Geometry: final body of the model. Coordinates: model frame, mm. A direction names the side the tool comes from. Give positions to 0.01 mm unless a question says otherwise; leave off trailing zeros. Write each loop counter-clockwise with the first axis right and the second up, starting at its lowest first coordinate (ties: lowest second). Pieces come first, ordered by that corner, then holes. Notation, with made-up numbers: M 67.5,-33.5 L 112.5,-33.5 A25 cw 112.5,1.5 Z; hole C -3,28 d11. An arc over 180 degrees is marked long. Use a Markdown table: item, result. Add a question column.
(1) Pin query (flat end, axial travel): pin 1 Ø1.5 at (y, z) = (-2, -14) entering from +X; pin 2 Ø1.5 at (x, y) = (-9.5, -1) entering from +Z; pin 3 Ø1.5 at (x, z) = (-1, -37.5) entering from -Y. Return the tip coordinate at first contact, or that it passes through.
(2) Cut plane C-C (z = -17.5). Output: boundary loops of the cut face in (x, y), plus the area to 3 significant figures.
(3) Cut plane A-A (x = -11.25). Output: boundary loops of the cut face in (y, z), plus the area to 3 significant figures.
(4) Reachability of faces 4 (the flat face through (-4, 3, -25)), 5 (the flat face through (5, 1, -20)), 6 (the flat face through (4, 0, -25)) from +Z, -Z, +X, -X, +Y, -Y: full face, straight path, thin tool, end or side. Return the list, or none.
(5) Cut plane D-D (x = 6.5). Output: boundary loops of the cut face in (y, z), plus the area to 3 significant figures.
(6) Material intervals for L1, parallel to Z at x = 6, y = 1.15; L2, parallel to X at y = 1.55, z = -43.5; L3, parallel to Z at x = -10.75, y = -1.9, sorted ascending.
(7) Cut plane B-B (y = -1.65). Output: boundary loops of the cut face in (x, z).
(8) Draft query along Z for faces 1 (the flat face through (-7, 1, -50)), 2 (the flat face through (-18, 0, -25)), 3 (the flat face through (5, 1, -42)). Return one class per face: released by +Z, released by -Z, zero draft, split by the parting line, or undercut.
Autodesk Inventor part; units mm, degrees
ref_plane "YZ Plane" through (0, 0, 0) normal (1, 0, 0) x (0, 1, 0)
ref_plane "XZ Plane" through (0, 0, 0) normal (0, 1, 0) x (-1, 0, 0)
ref_plane "XY Plane" through (0, 0, 0) normal (0, 0, 1) x (1, 0, 0)
sketch "Sketch1" plane through (0, 0, 0) normal (0, 1, 0) x (-1, 0, 0)
  line L0 (0, 0) -> (0, -50)
  line L1 (0, -50) -> (-10, -50)
  line L2 (-10, -50) -> (-10, 0)
  line L3 (-10, 0) -> (0, 0)
  line L4 (-5, -50) -> (-5, -46)
  line L5 (-5, -46) -> (-3, -46)
  line L6 (-3, -46) -> (-3, -42)
  line L7 (-3, -42) -> (-7, -42)
  line L8 (-7, -42) -> (-7, -46)
  line L9 (-7, -46) -> (-5, -46)
  line L10 (-5, -42) -> (-5, -33)
  line L11 (-5, -33) -> (-7, -33)
  line L12 (-7, -33) -> (-7, -29)
  line L13 (-7, -29) -> (-3, -29)
  line L14 (-3, -29) -> (-3, -33)
  line L15 (-5, -33) -> (-3, -33)
  line L16 (-5, -29) -> (-5, -20)
  line L17 (-5, -20) -> (-3, -20)
  line L18 (-3, -20) -> (-3, -16)
  line L19 (-3, -16) -> (-7, -16)
  line L20 (-7, -16) -> (-7, -20)
  line L21 (-5, -20) -> (-7, -20)
  line L22 (-5, -16) -> (-5, -7)
  line L23 (-5, -7) -> (-7, -7)
  line L24 (-7, -7) -> (-7, -3)
  line L25 (-7, -3) -> (-3, -3)
  line L26 (-5, -7) -> (-3, -7)
  line L27 (-3, -7) -> (-3, -3)
  line L28 (0, -50) -> (2, -50)
  line L29 (2, -50) -> (2, 0)
  line L30 (2, 0) -> (0, 0)
  dimension "d0" = 50
  dimension "d1" = 10
  dimension "d2" = 90
  dimension "d3" = 4
  dimension "d4" = 2
  dimension "d5" = 4
  dimension "d6" = 4
  dimension "d7" = 9
  dimension "d8" = 4
  dimension "d9" = 9
  dimension "d10" = 4
  dimension "d11" = 9
  dimension "d12" = 4
  dimension "d13" = 2
extrude "Extrusion1" add sketch "Sketch1" along normal blind 3
sketch "Sketch2" plane through (-2, 0, -50) normal (-1, 0, 0) x (0, 0, 1)
  line L0 (0, 0) -> (0, 3)
  line L1 (0, 3) -> (50, 3)
  line L2 (50, 3) -> (50, -3)
  line L3 (50, -3) -> (0, -3)
  line L4 (0, -3) -> (0, 3)
  point P0 (50, 0)
  dimension "d16" = 6
extrude "Extrusion2" add sketch "Sketch2" along normal blind 16
sketch "Sketch3" plane through (0, 3, 0) normal (0, 1, 0) x (1, 0, 0)
  line L0 (-2, 0) -> (-18, 0)
  line L1 (-10, 0) -> (-10, 50)
  line L2 (10, 50) -> (-18, 50)
  line L3 (-12.5, 41.5) -> (-7.5, 41.5)
  line L4 (-7.5, 41.5) -> (-7.5, 46.5)
  line L5 (-7.5, 46.5) -> (-12.5, 46.5)
  line L6 (-12.5, 46.5) -> (-12.5, 41.5)
  line L7 (-12.5, 41.5) -> (-7.5, 46.5) construction
  line L8 (-7.5, 41.5) -> (-12.5, 46.5) construction
  line L9 (-12.5, 2.5) -> (-7.5, 2.5)
  line L10 (-7.5, 2.5) -> (-7.5, 7.5)
  line L11 (-7.5, 7.5) -> (-12.5, 7.5)
  line L12 (-12.5, 7.5) -> (-12.5, 2.5)
  line L13 (-12.5, 2.5) -> (-7.5, 7.5) construction
  line L14 (-7.5, 2.5) -> (-12.5, 7.5) construction
  line L15 (-12, 16) -> (-8, 16)
  line L16 (-8, 16) -> (-8, 20)
  line L17 (-8, 20) -> (-12, 20)
  line L18 (-12, 20) -> (-12, 16)
  line L19 (-12, 16) -> (-8, 20) construction
  line L20 (-8, 16) -> (-12, 20) construction
  line L21 (-12.25, 28.75) -> (-7.75, 28.75)
  line L22 (-7.75, 28.75) -> (-7.75, 33.25)
  line L23 (-7.75, 33.25) -> (-12.25, 33.25)
  line L24 (-12.25, 33.25) -> (-12.25, 28.75)
  line L25 (-12.25, 28.75) -> (-7.75, 33.25) construction
  line L26 (-7.75, 28.75) -> (-12.25, 33.25) construction
  point P0 (0, 0)
  point P1 (-10, 44)
  point P2 (-10, 5)
  point P3 (-10, 18)
  point P4 (-10, 31)
  dimension "d19" = 5
  dimension "d20" = 5
  dimension "d21" = 5
  dimension "d22" = 5
  dimension "d23" = 4
  dimension "d24" = 4
  dimension "d25" = 4.5
  dimension "d26" = 4.5
extrude "Extrusion3" cut sketch "Sketch3" against normal blind 16
sketch "Sketch4" plane through (-2, -3, -50) normal (0, -1, 0) x (1, 0, 0)
  point P0 (2, 50)
equation "\"BendRadius\" = Thickness"
equation "\"BendReliefWidth\" = Thickness"
equation "\"BendReliefDepth\" = 0.5 * Thickness"
equation "\"CornerReliefSize\" = 4 * Thickness"
equation "\"MinimumRemnant\" = 2 * Thickness"
equation "\"TransitionRadius\" = BendRadius"
equation "\"JacobiRadiusSize\" = BendRadius"
equation "\"GapSize\" = Thickness"
Answer list:
| question | item | result |
|---|---|---|
| 1 | pin 1 | x = -2 |
| 1 | pin 2 | z = 0 |
| 1 | pin 3 | y = 0 |
| 2 | outline | M -18,-3 L -12,-3 L -12,3 L -18,3 Z; M -8,-3 L -2,-3 L -2,0 L 3,0 L 3,3 L -8,3 Z; M 7,0 L 10,0 L 10,3 L 7,3 Z |
| 2 | area | 96.0 mm² |
| 3 | outline | M -3,-50 L 3,-50 L 3,-46.5 L -3,-46.5 Z; M -3,-41.5 L 3,-41.5 L 3,-33.25 L -3,-33.25 Z; M -3,-28.75 L 3,-28.75 L 3,-20 L -3,-20 Z; M -3,-16 L 3,-16 L 3,-7.5 L -3,-7.5 Z; M -3,-2.5 L 3,-2.5 L 3,0 L -3,0 Z |
| 3 | area | 189 mm² |
| 4 | face 4 | +Z, -Z, +X, -X, +Y |
| 4 | face 5 | +Y, -Y |
| 4 | face 6 | +Z, -Z, +X, -Y |
| 5 | outline | M 0,-50 L 3,-50 L 3,-46 L 0,-46 Z; M 0,-42 L 3,-42 L 3,-33 L 0,-33 Z; M 0,-29 L 3,-29 L 3,-20 L 0,-20 Z; M 0,-16 L 3,-16 L 3,-7 L 0,-7 Z; M 0,-3 L 3,-3 L 3,0 L 0,0 Z |
| 5 | area | 102 mm² |
| 6 | L1 | -50 to -46, -42 to -33, -29 to -20, -16 to -7, -3 to 0 |
| 6 | L2 | -18 to -12.5, -7.5 to 3, 7 to 10 |
| 6 | L3 | -50 to -46.5, -41.5 to -33.25, -28.75 to -20, -16 to -7.5, -2.5 to 0 |
| 7 | outline | M -18,-50 L -2,-50 L -2,0 L -18,0 Z; hole M -12.5,-46.5 L -7.5,-46.5 L -7.5,-41.5 L -12.5,-41.5 Z; hole M -12.5,-7.5 L -7.5,-7.5 L -7.5,-2.5 L -12.5,-2.5 Z; hole M -12.25,-33.25 L -7.75,-33.25 L -7.75,-28.75 L -12.25,-28.75 Z; hole M -12,-20 L -8,-20 L -8,-16 L -12,-16 Z |
| 8 | face 1 | released by -Z |
| 8 | face 2 | zero draft |
| 8 | face 3 | undercut |
